Design review of the part built by this model. Coordinates are the model's own, in mm. Give positions to 0.01 mm unless a question says otherwise; leave off trailing zeros. Loops run counter-clockwise (first coordinate to the right, second up) from the corner with the lowest first, then second, coordinate; pieces in that order, holes last. Notation, with made-up numbers: (80.5, 22.5) - (130.5, 22.5) arc R19 cw to (130.5, 49.5) - close; hole circle Ø11 at (18.25, 35.25). An arc over 180 degrees is marked (long way). One line per item, written item: value. Start each with the question number.
```python
from build123d import *

# Parameters (mm, degrees)
SKETCH_1_R          = 3
EXTRUDE_2_DEPTH     = 2.5
SKETCH_4_OUTSIDE_W  = 48.83
SKETCH_4_OUTSIDE_H  = 46.628
SKETCH_4_OUTSIDE_R  = 7.116873297
CUT_EXTRUDE_1_DEPTH = 12.965912678
CUT_EXTRUDE_1_DRAFT = -45
SKETCH_5_OUTSIDE_W  = 48.83
SKETCH_5_OUTSIDE_H  = 46.628
SKETCH_5_OUTSIDE_R  = 7.116873297
CUT_EXTRUDE_2_DEPTH = 12.965912678
CUT_EXTRUDE_2_DRAFT = -45


with BuildPart() as part:
    # 草图1 → 凸台-拉伸2 (new, symmetric)
    with BuildSketch(Plane(origin=(0, 0, 0), x_dir=(1, 0, 0), z_dir=(0, 1, 0))):
        Polygon((8.217857428, 0), (4.108928714, 7.116873297), (-4.108928714, 7.116873297), (-8.217857428, 0), (-4.108928714, -7.116873297), (4.108928714, -7.116873297), align=None)
        with Locations(Location((0, 0, 0), (0, 0, 270))):
            Circle(SKETCH_1_R, mode=Mode.SUBTRACT)
    extrude(amount=EXTRUDE_2_DEPTH, both=True)


with BuildPart() as cut_extrude_1_tool:
    # 草图4 outside → 切除-拉伸1 (with draft: the straight prism first)
    with BuildSketch(Plane(origin=(0, 2.5, 0), x_dir=(1, 0, 0), z_dir=(0, 1, 0))):
        Rectangle(SKETCH_4_OUTSIDE_W, SKETCH_4_OUTSIDE_H)
        Circle(SKETCH_4_OUTSIDE_R, mode=Mode.SUBTRACT)
    extrude(amount=-CUT_EXTRUDE_1_DEPTH)
    # 切除-拉伸1: the draft: its side faces are tilted about the plane it starts from
    cut_extrude_1_sides = [cut_extrude_1_tool.faces().sort_by_distance(p)[0] for p in [
        (0, -3.982956339, 23.314),
        (24.415, -3.982956339, 0),
        (0, -3.982956339, -23.314),
        (-24.415, -3.982956339, 0),
        (-7.116873297, -3.982956339, 0),
    ]]
    draft(cut_extrude_1_sides, Plane(origin=(0, 2.5, 0), x_dir=(1, 0, 0), z_dir=(0, 1, 0)), CUT_EXTRUDE_1_DRAFT)


with BuildPart() as part_1:
    add(part.part)

    # 切除-拉伸1: cut by cut_extrude_1_tool
    add(cut_extrude_1_tool.part, mode=Mode.SUBTRACT)


with BuildPart() as cut_extrude_2_tool:
    # 草图5 outside → 切除-拉伸2 (with draft: the straight prism first)
    with BuildSketch(Plane.XZ.offset(2.5)):
        Rectangle(SKETCH_5_OUTSIDE_W, SKETCH_5_OUTSIDE_H)
        Circle(SKETCH_5_OUTSIDE_R, mode=Mode.SUBTRACT)
    extrude(amount=-CUT_EXTRUDE_2_DEPTH)
    # 切除-拉伸2: the draft: its side faces are tilted about the plane it starts from
    cut_extrude_2_sides = [cut_extrude_2_tool.faces().sort_by_distance(p)[0] for p in [
        (0, 3.982956339, -23.314),
        (24.415, 3.982956339, 0),
        (0, 3.982956339, 23.314),
        (-24.415, 3.982956339, 0),
        (-7.116873297, 3.982956339, 0),
    ]]
    draft(cut_extrude_2_sides, Plane.XZ.offset(2.5), CUT_EXTRUDE_2_DRAFT)


with BuildPart() as part_2:
    add(part_1.part)

    # 切除-拉伸2: cut by cut_extrude_2_tool
    add(cut_extrude_2_tool.part, mode=Mode.SUBTRACT)


solid = part_2.part
```
(1) Take a section at B-B on y = 1.6. State the section outline as (x, z) points.
(2) Draft analysis for pull direction X (two halves, no side actions). For faces 1 (the cylindrical face through (0.9, -0.04, 2.86)), 2 (the conical face through (-7.379, 2.238, -0.018)), 3 (the conical face through (3.705, 2.238, -6.382)), state which applies: pulls with the +X half, pulls with the -X half, needs draft (parallel to the pull), parting line crosses it, or undercut.
(3) To check wall thickness, follow L1, parallel to X at y = -1.65, z = -0.75; L2, parallel to Z at x = -0.5, y = 0.2; L3, parallel to X at y = 1.4, z = 2. State the ranges of each line that lie inside material, in increasing order. Write a range as from..to.
(4) Take a section at A-A on y = -0.8. State the section outline as (x, z) points, and give its area (3 significant figures).
(5) For pin 1 Ø3 at (y, z) = (0, -5.5) entering from -X; pin 2 Ø1 at (y, z) = (-0.5, 5) entering from -X, all flat-tipped, find the tip position at first contact; note any pin that passes through.
Here are the results:
1. outline: (-8.01, -0.36) - (-4.32, -6.75) arc R8.02 ccw to (-3.69, -7.12) - (3.69, -7.12) arc R8.02 ccw to (4.32, -6.75) - (8.01, -0.36) arc R8.02 ccw to (8.01, 0.36) - (4.32, 6.75) arc R8.02 ccw to (3.69, 7.12) - (-3.69, 7.12) arc R8.02 ccw to (-4.32, 6.75) - (-8.01, 0.36) arc R8.02 ccw to start; hole circle Ø6 at (0, 0)
2. face 1: undercut
2. face 2: pulls with the -X half
2. face 3: pulls with the +X half
3. L1: -7.78..-2.9, 2.9..7.78
3. L2: -7.12..-2.96, 2.96..7.12
3. L3: -7.06..-2.24, 2.24..7.06
4. outline: (-8.22, 0) - (-4.11, -7.12) - (4.11, -7.12) - (8.22, 0) - (4.11, 7.12) - (-4.11, 7.12) - close; hole circle Ø6 at (0, 0)
4. area: 147 mm²
5. pin 1: x = -5.91
5. pin 2: x = -5.62
